Could you check a few things on this model? Use its own coordinates, in mm. A direction names the side the tool comes from. Give positions to 0.01 mm unless a question says otherwise; leave off trailing zeros. Write each loop counter-clockwise with the first axis right and the second up, starting at its lowest first coordinate (ties: lowest second). Pieces come first, ordered by that corner, then holes. Notation, with made-up numbers: M 11.25,47 L 65.25,47 A17 ccw 65.25,65 Z; hole C 86.25,80.25 d8. An arc over 180 degrees is marked long. One line per item, written item: value.
```python
from build123d import *

# Parameters (mm, degrees)
BOSS_EXTRUDE2_DEPTH     = 40
BOSS_EXTRUDE2_2_DEPTH   = 40
BOSS_EXTRUDE3_START     = -1
BOSS_EXTRUDE3_DEPTH     = 1
FILLET1_R               = 1
FILLET2_R               = 5
CUT_EXTRUDE1_DEPTH      = 85.5295373443375
CUT_EXTRUDE1_DEPTH_BACK = 85.5295373443375
SKETCH4_R               = 1.5000000000000004
SKETCH4_R_2             = 1.5000000000000009
SKETCH4_R_3             = 1.4999999999999991
CUT_EXTRUDE2_DEPTH      = 1


with BuildPart() as part:
    # Sketch1 → Boss-Extrude2 (new body)
    with BuildSketch(Plane(origin=(0, 0, 0), x_dir=(1, 0, 0), z_dir=(0, 1, 0))):
        with BuildLine():
            Line((-25.401627045652027, 65.22850100556965), (-10, 22.912878474779202))
            ThreePointArc((-10.000000000000004, 22.912878474779205), (-9.53932578125167, 23.108467358073476), (-9.0748285709005, 23.294795264366854))
            Line((-9.074828570900502, 23.294795264366854), (-24.46711558509191, 65.58475626962223))
            ThreePointArc((-24.46711558509193, 65.58475626962225), (-24.935007566594734, 65.40829762082075), (-25.401627045652038, 65.22850100556964))
        make_face()
    extrude(amount=BOSS_EXTRUDE2_DEPTH)



with BuildPart() as body_2:
    # Sketch1 → Boss-Extrude2 2 (new body)
    with BuildSketch(Plane(origin=(0, 0, 0), x_dir=(1, 0, 0), z_dir=(0, 1, 0))):
        with BuildLine():
            Line((24.46711558509189, 65.58475626962225), (9.074828570900499, 23.294795264366847))
            ThreePointArc((9.0748285709005, 23.294795264366854), (9.53932578125167, 23.108467358073483), (10, 22.912878474779205))
            Line((10, 22.912878474779205), (25.401627045652017, 65.22850100556967))
            ThreePointArc((25.401627045652017, 65.22850100556967), (24.935007566594702, 65.40829762082078), (24.467115585091896, 65.58475626962228))
        make_face()
    extrude(amount=BOSS_EXTRUDE2_2_DEPTH)


with BuildPart() as part_1:
    add(part.part)

    add(body_2.part)  # Boss-Extrude3 merges body 2
    # Sketch1<5> → Boss-Extrude3 (add)
    with BuildSketch(Plane(origin=(0, 0, 0), x_dir=(1, 0, 0), z_dir=(0, 1, 0)).offset(BOSS_EXTRUDE3_START)):
        with BuildLine():
            Line((-25.401627045652027, 65.22850100556965), (-10, 22.912878474779202))
            ThreePointArc((-10, 22.912878474779205), (-8.9e-16, 25), (9.999999999999996, 22.912878474779205))
            Line((10, 22.912878474779205), (25.401627045652017, 65.22850100556967))
            ThreePointArc((25.401627045652017, 65.22850100556967), (-1.421e-14, 70.00000000000003), (-25.401627045652038, 65.22850100556964))
        make_face()
    extrude(amount=BOSS_EXTRUDE3_DEPTH)

    # Fillet1
    fillet1_edges = [part_1.edges().sort_by_distance(p)[0] for p in [
        (16.770972077996195, 0, -44.43977576699454),
        (-16.770972077996205, 0, -44.43977576699454),
    ]]
    fillet(fillet1_edges, radius=FILLET1_R)

    # Fillet2
    # the kernel refuses this fillet: 5 mm, written as the material it takes off along each edge
    with BuildSketch(Plane(origin=(4.656364e-11, 40, 1.1895196e-10), x_dir=(-0.1775518542225804, 0, -0.9841114464643339), z_dir=(0.9841114464643339, 0, -0.1775518542225804))) as fillet2_piece_1:
        with BuildLine():
            CenterArc((70.00000000012774 - FILLET2_R, -FILLET2_R), FILLET2_R, 0, 90)
            Line((70.00000000012774 - FILLET2_R, 0), (70.00000000012774, 0))
            Line((70.00000000012774, 0), (70.00000000012774, -FILLET2_R))
        make_face()
    revolve(axis=Axis((4.656364e-11, 40, 1.1895196e-10), (0, 1, 0)), revolution_arc=21.281391087786062, mode=Mode.SUBTRACT)
    with BuildSketch(Plane(origin=(-2.019185e-11, 40, 5.042011e-11), x_dir=(0.5226263256133499, 0, -0.8525618592078166), z_dir=(0.8525618592078166, 0, 0.5226263256133499))) as fillet2_piece_2:
        with BuildLine():
            CenterArc((70.00000000010422 - FILLET2_R, -FILLET2_R), FILLET2_R, 0, 89.99999999999983)
            Line((70.00000000010422 - FILLET2_R, 0), (70.00000000010422, 0))
            Line((70.00000000010422, 0), (70.00000000010421, -FILLET2_R))
        make_face()
    revolve(axis=Axis((-2.019185e-11, 40, 5.042011e-11), (0, 1, 0)), revolution_arc=21.281391087808515, mode=Mode.SUBTRACT)

    # Sketch3 → Cut-Extrude1 (cut, two sides: drawn at the far end of the back side and taken through both)
    with BuildSketch(Plane(origin=(0, 0, 0), x_dir=(0, 0, -1), z_dir=(1, 0, 0)).offset(-CUT_EXTRUDE1_DEPTH_BACK)):
        Polygon((22.912878474779205, 13.999999999999998), (37.92398547370926, 40), (22.912878474779205, 40), (17.723420287047986, 40), (17.723420287047986, 13.999999999999998), align=None)
    extrude(amount=CUT_EXTRUDE1_DEPTH + CUT_EXTRUDE1_DEPTH_BACK, mode=Mode.SUBTRACT)

    # Sketch4 → Cut-Extrude2 (cut)
    with BuildSketch(Plane(origin=(0, 0, 0), x_dir=(1, 0, 0), z_dir=(0, 1, 0))):
        with Locations(Location((2.4e-16, 40, 0), (0, 0, 270))):
            Circle(SKETCH4_R)
        with Locations(Location((-15.529142706151296, 57.95554957734408, 0), (0, 0, 270))):
            Circle(SKETCH4_R_2)
        with Locations(Location((15.529142706151275, 57.955549577344094, 0), (0, 0, 270))):
            Circle(SKETCH4_R_3)
    extrude(amount=-CUT_EXTRUDE2_DEPTH, mode=Mode.SUBTRACT)


solid = part_1.part
```
1) I'm going to push flat-ended pins straight in: pin 1 (2 mm diameter, centred on y = 20.5, z = -37, fed in from +X); pin 2 (5 mm diameter, centred on y = 21.5, z = -30.5, fed in from +X); pin 3 (1.5 mm diameter, centred on x = 15.5, z = -55, fed in from +Y). Where does each tip first touch, or does it pass through?
Outcome:
pin 1: stops at x = 15.49
pin 2: stops at x = 13.67
pin 3: stops at y = 0
2) Please list where these lines run through material, in increasing order: L1, parallel to Y at x = -1, z = -57; L2, parallel to X at y = 25.5, z = -43.5; L3, parallel to X at y = 2, z = -45.5. Write a range as from..to.
Outcome:
L1: y = -1..0
L2: x = -17.49..-16.43, 16.43..17.49
L3: x = -18.22..-17.16, 17.16..18.22
3) We'd pull the mould along X, two halves only. Please class faces 3 (the face through (11.62, -0.42, -69.03)), 4 (the face through (0, -0.2, -25)), 5 (the face through (15.595, -0.493, -59.454)), 6 (the face through (-12.284, 26.939, -30.383)): pulls with the +X half, pulls with the -X half, needs draft (parallel to the pull), parting line crosses it, or undercut.
Outcome:
face 3: parting line crosses it
face 4: undercut
face 5: undercut
face 6: needs draft
4) If we section it at B-B, the plane y = 6.5: Write out the boundary of the cut face in (x, z).
Outcome:
outline: M -25.4,-65.23 A70 ccw -24.47,-65.58 L -9.07,-23.29 A25 cw -10,-22.91 Z; M 9.07,-23.29 L 24.47,-65.58 A70 ccw 25.4,-65.23 L 10,-22.91 A25 cw Z
5) If we section it at A-A, the plane x = 0: Write out the boundary of the cut face in (y, z), then the cut area to 3 significant figures.
Outcome:
outline: M -1,-70 L 0,-70 L 0,-41.5 L -1,-41.5 Z; M -1,-38.5 L 0,-38.5 L 0,-25 L -1,-25 Z
area: 42.0 mm^2
6) On a 3-axis mill with a long thin cutter (end or side, diameter ignored), from which of +Z, -Z, +X, -X, +Y, -Y can I reach the whole of each face in a straight line? I mean faces 1 (the face through (-16.66, 20.23, -44.14)), 2 (the face through (-19, 40, -49)). Say none if no direction works.
Outcome:
face 1: -Z, +Y
face 2: +Z, -Z, +X, -X, +Y
